Here's the drawing with two shaded views (mm, measured from the low corner). I have some questions. A direction names the side the tool comes from. Coordinates: 2 decimals unless noted, no trailing zeros. Order: outer loops, then holes, each group sorted by start corner. A loop starts at its lowest first (then second) coordinate and runs counter-clockwise, first axis right, second up. Notation, with made-up numbers: (45, -0.75) - (68, -0.75) arc R30 ccw to (68, 24.25) - close; hole circle Ø6 at (-5.75, 78). An arc over 180 degrees is marked (long way). Answer as a JSON object with one key per item and string values. Group by question number.
(1) Imagine slicing it at A-A, the plane y = 15. Write out the boundary of the cut face in (x, z).
(2) Please list where these lines run through material, in increasing order: probe 1 along Y at (x, z) = (130, 102); probe 2 along Y at (x, z) = (95, 103.5); probe 3 along X at (y, z) = (15, 102).
(3) Will this pin go through, and if not, where does the flat tip stop? P1, Ø1, axis at x = 154.5, y = 58, coming from the -Z side.
(4) Imagine slicing it at C-C, the plane z = 18. Write out the boundary of the cut face in (x, y).
(5) We'd pull the mould along X, two halves only. Please class the marked faces 3, 4, 5 and 6: pulls with the +X half, pulls with the -X half, needs draft (parallel to the pull), parting line crosses it, or undercut.
(6) Which directions (+Z, -Z, +X, -X, +Y, -Y) give clear straight access to the entire face, cutting with the end or side of a thin tool? Please do the marked faces 1 and 2.
(7) Imagine slicing it at B-B, the plane x = 60. Write out the boundary of the cut face in (y, z).
(8) Imagine slicing it at D-D, the plane y = 50. Write out the boundary of the cut face in (x, z).
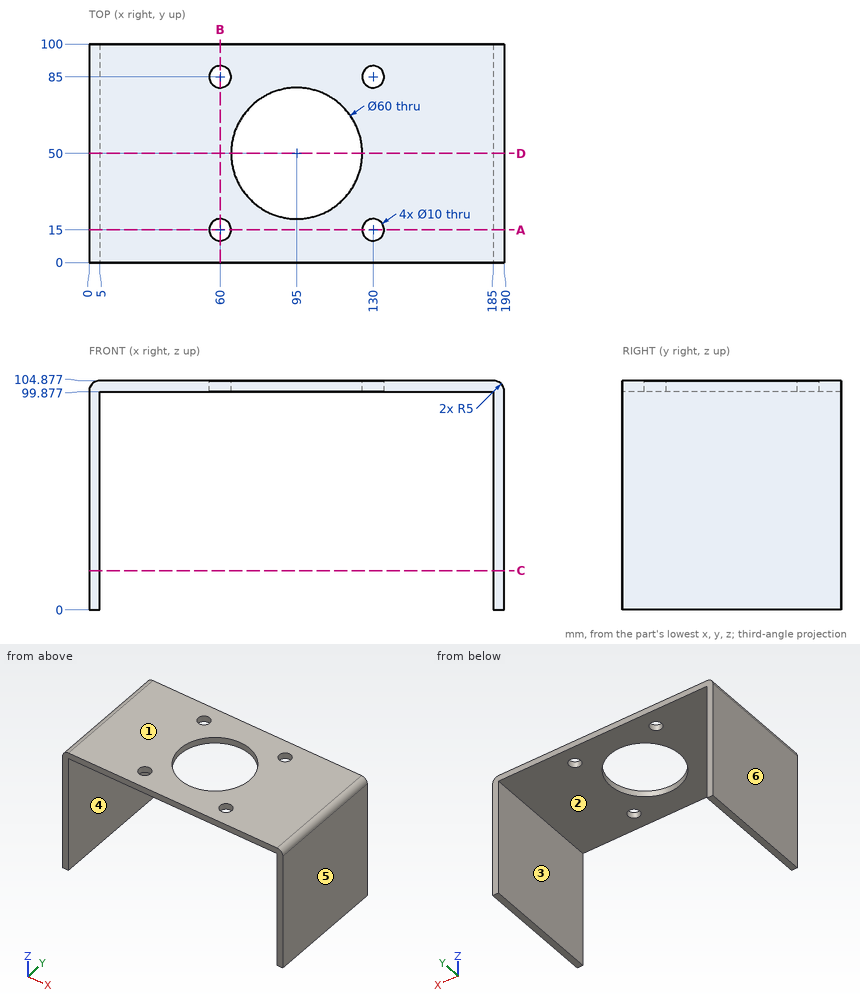
Result set:
{
 "1": {"outline": "(0, 0) - (5, 0) - (5, 99.88) - (55, 99.88) - (55, 104.88) - (5, 104.88) arc R5 ccw to (0, 99.88) - close; (65, 99.88) - (125, 99.88) - (125, 104.88) - (65, 104.88) - close; (135, 99.88) - (185, 99.88) - (185, 0) - (190, 0) - (190, 99.88) arc R5 ccw to (185, 104.88) - (135, 104.88) - close"},
 "2": {"probe 1": "y = 0 to 10, 20 to 80, 90 to 100", "probe 2": "y = 0 to 20, 80 to 100", "probe 3": "x = 0.47 to 55, 65 to 125, 135 to 189.53"},
 "3": {"P1": "stops at z = 99.88"},
 "4": {"outline": "(0, 0) - (5, 0) - (5, 100) - (0, 100) - close; (185, 0) - (190, 0) - (190, 100) - (185, 100) - close"},
 "5": {"face 3": "undercut", "face 4": "undercut", "face 5": "pulls with the +X half", "face 6": "pulls with the -X half"},
 "6": {"face 1": "+Z, +X, -X, +Y, -Y", "face 2": "-Z, +Y, -Y"},
 "7": {"outline": "(0, 99.88) - (10, 99.88) - (10, 104.88) - (0, 104.88) - close; (20, 99.88) - (80, 99.88) - (80, 104.88) - (20, 104.88) - close; (90, 99.88) - (100, 99.88) - (100, 104.88) - (90, 104.88) - close"},
 "8": {"outline": "(0, 0) - (5, 0) - (5, 99.88) - (65, 99.88) - (65, 104.88) - (5, 104.88) arc R5 ccw to (0, 99.88) - close; (125, 99.88) - (185, 99.88) - (185, 0) - (190, 0) - (190, 99.88) arc R5 ccw to (185, 104.88) - (125, 104.88) - close"}
}
